```python
from build123d import *

# Parameters (mm, degrees)
F0_R     = 6.434371
F0_R_2   = 7.574086
F1_DEPTH = 25.4
F2_W     = 3.636818
F2_H     = 3.357063
F2_W_2   = 13.428252
F2_W_3   = 5.315348
F3_DEPTH = 25.4


with BuildPart() as f1:
    # F0 (on Front) → F1 (new body)
    with BuildSketch(Plane.XZ):
        with BuildLine():
            ThreePointArc((-16.227132, 24.940537), (-14.186517, -26.15517), (29.754834, 0))
            ThreePointArc((29.754834, 0), (22.887437, 19.013558), (5.455228, 29.250481))
            ThreePointArc((5.455228, 29.250481), (1.427673, 29.720564), (-2.626396, 29.638695))
            ThreePointArc((-2.626396, 29.638695), (-5.634264, 29.216524), (-8.583421, 28.489912))
            ThreePointArc((-8.583421, 28.489912), (-12.531576, 26.987215), (-16.227132, 24.940537))
        make_face()
        with Locations((-12.449108, 13.847885)):
            Circle(F0_R, mode=Mode.SUBTRACT)
        with Locations((11.050331, 13.847885)):
            Circle(F0_R_2, mode=Mode.SUBTRACT)
        with BuildLine():
            ThreePointArc((-2.626396, 29.638695), (1.427673, 29.720564), (5.455228, 29.250481))
            Line((5.455228, 29.250481), (5.455228, 45.698488))
            Line((5.455228, 45.698488), (-2.626396, 45.698488))
            Line((-2.626396, 45.698488), (-2.626396, 29.638695))
        make_face()
        with BuildLine():
            Line((-26.436771, 41.263932), (-16.227132, 24.940537))
            ThreePointArc((-16.227132, 24.940537), (-12.531576, 26.987215), (-8.583421, 28.489912))
            Line((-8.583421, 28.489912), (-19.346706, 45.698488))
            Line((-19.346706, 45.698488), (-26.436771, 41.263932))
        make_face()
    extrude(amount=F1_DEPTH)

    # F2 (on Front) → F3 (join)
    with BuildSketch(Plane.XZ):
        with Locations((-8.112902, -10.770577)):
            Rectangle(F2_W, F2_H)
        with Locations((0.419633, -10.770577)):
            Rectangle(F2_W_2, F2_H)
        with Locations((9.791433, -10.770577)):
            Rectangle(F2_W_3, F2_H)
        Polygon((0, 0), (0, 11.609843), (-7.13376, 0), align=None)
    extrude(amount=F3_DEPTH)


solid = f1.part
```
Design review of the part built by this model. Coordinates are the model's own, in mm. A direction names the side the tool comes from. Round coordinates to 2 decimals unless told otherwise and drop trailing zeros. Write each loop counter-clockwise with the first axis right and the second up, starting at its lowest first coordinate (ties: lowest second). Pieces come first, ordered by that corner, then holes. Notation, with made-up numbers: (5.25, -37) -> (47.25, -37) arc R27 cw to (47.25, -7) -> close; hole circle Ø10 at (18, 63). An arc over 180 degrees is marked (long way). Write item = value, one per line. Start each with the question number.
1) Tool access review of faces 5 (the face through (1, -13, 45.698)), 6 (the face through (-5.592, -12.522, 29.225)): name each direction out of +Z, -Z, +X, -X, +Y, -Y from which nothing blocks a thin tool from reaching the whole face with its end or side.
2) Wall thickness on probe 1 along Z at (x, y) = (0, -21.75); probe 2 along X at (y, z) = (-6.25, 8.5); probe 3 along Z at (x, y) = (-18, -20.25): over which ranges is each line inside the solid? List them lowest first. Write a range as from..to.
3) Take a section at C-C, the plane x = -15. State the section outline as (y, z) points (3 decimals), plus the area to 3 significant figures.
4) Clearance check with flat-ended pins moving along their axes: pin 1 (1 mm diameter, centred on y = -4, z = -6, fed in from +X); pin 2 (1.5 mm diameter, centred on y = -4.5, z = 36.5, fed in from -X); pin 3 (5 mm diameter, centred on y = -16, z = 37, fed in from +X). State where each tip first meets the part, or that it passes through.
5) Take a section at B-B, the plane y = -16.5. State the section outline as (x, z) points.
6) Take a section at D-D, the plane z = -7.5. State the section outline as (x, y) points, plus the area to 3 significant figures.
7) Mouldability with a two-part tool opening along Z and no side actions: class faces 1 (the face through (5.455, -13, 37)), 2 (the face through (-21.403, -12.522, 33.216)), 3 (the face through (-6.5, -12.5, 11.4)), 4 (the face through (-22.842, -12.522, 43.512)) as +Z half, -Z half, draft (parallel to the pull), parting line (faces both ways), or undercut.
8) Take a section at A-A, the plane x = -22. State the section outline as (y, z) points.
Results list:
q1.face_5 = +Z, +X, -X, +Y, -Y
q1.face_6 = +Z, +Y, -Y
q2.probe_1 = -29.75..45.7
q2.probe_2 = -28.51..-16.03, -8.87..5.69, 16.41..28.51
q2.probe_3 = -23.69..10.59, 17.1..23.69, 27.78..43.55
q3.outline = (-25.4, -25.697) -> (0, -25.697) -> (0, 7.941) -> (-25.4, 7.941) -> close; (-25.4, 19.755) -> (0, 19.755) -> (0, 38.749) -> (-25.4, 38.749) -> close
q3.area = 1,340 mm²
q4.pin_1 = 29.24
q4.pin_2 = -23.93
q4.pin_3 = 5.46
q5.outline = (-26.44, 41.26) -> (-16.23, 24.94) arc R29.75 ccw (long way) to (29.75, 0) arc R29.75 ccw to (5.46, 29.25) -> (5.46, 45.7) -> (-2.63, 45.7) -> (-2.63, 29.64) arc R29.75 ccw to (-8.58, 28.49) -> (-19.35, 45.7) -> close; hole circle Ø12.87 at (-12.45, 13.85); hole circle Ø15.15 at (11.05, 13.85)
q6.outline = (-28.79, -25.4) -> (28.79, -25.4) -> (28.79, 0) -> (-28.79, 0) -> close
q6.area = 1,460 mm²
q7.face_1 = draft
q7.face_2 = undercut
q7.face_3 = undercut
q7.face_4 = +Z half
q8.outline = (-25.4, -20.03) -> (0, -20.03) -> (0, 20.03) -> (-25.4, 20.03) -> close; (-25.4, 34.17) -> (0, 34.17) -> (0, 44.04) -> (-25.4, 44.04) -> close
